```python
from build123d import *

# Parameters (mm, degrees)
SKETCH1_W            = 90
SKETCH1_H            = 120
BOSS_EXTRUDE1_DEPTH  = 15
SKETCH2_W            = 46
SKETCH2_H            = 30
CUT_EXTRUDE1_DEPTH   = 12
SKETCH3_W            = 44
SKETCH3_H            = 30
CUT_EXTRUDE2_DEPTH   = 8
SHELL1_START         = -47.6
SHELL1_OUTLINE_W     = 85.2
SHELL1_OUTLINE_H     = 13
SHELL1_DEPTH         = 45.2
SHELL1_START_2       = -117.6
SHELL1_2_OUTLINE_W   = 85.2
SHELL1_2_OUTLINE_H   = 5
SHELL1_2_DEPTH       = 35.2
SKETCH7_W            = 39
SKETCH7_H            = 34.8
CUT_EXTRUDE6_DEPTH   = 5
SKETCH11_W           = 42.056152249
SKETCH11_H           = 30
CUT_EXTRUDE9_DEPTH   = 2
CUT_EXTRUDE7_DEPTH   = 10
CUT_EXTRUDE10_DEPTH  = 3
SKETCH14_W           = 90
SKETCH14_H           = 120
SKETCH14_W_2         = 88.2
SKETCH14_H_2         = 118.2
BOSS_EXTRUDE2_DEPTH  = 1
SKETCH22_W           = 4
SKETCH22_H           = 30
BOSS_EXTRUDE6_DEPTH  = 8
SKETCH26_W           = 4
SKETCH26_H           = 12
CUT_EXTRUDE20_DEPTH  = 3.8
SKETCH27_R           = 1
CUT_EXTRUDE21_DEPTH  = 3
BOSS_EXTRUDE9_DEPTH  = 1.5
SKETCH40_R           = 3.5
CUT_EXTRUDE24_DEPTH  = 5
FILLET1_R            = 3
SKETCH44_W           = 85.2
SKETCH44_H           = 35.2
CUT_EXTRUDE25_DEPTH  = 7.8
SKETCH46_W           = 4.8
SKETCH46_H           = 15.6
BOSS_EXTRUDE15_DEPTH = 12.5
SKETCH6_R            = 0.9
CUT_EXTRUDE26_DEPTH  = 29.4
SKETCH47_W           = 33.8
SKETCH47_H           = 8
SKETCH47_W_2         = 8
BOSS_EXTRUDE16_DEPTH = 12.5
SKETCH49_W           = 41.022368698
SKETCH49_H           = 10
SKETCH49_W_2         = 8
BOSS_EXTRUDE17_DEPTH = 12.7
SKETCH50_W           = 22
SKETCH50_H           = 7
SKETCH50_W_2         = 20
SKETCH50_H_2         = 9
CUT_EXTRUDE28_DEPTH  = 12.5
FILLET3_R            = 5
FILLET4_R            = 2
SKETCH51_R           = 2.5
CUT_EXTRUDE29_DEPTH  = 6
CUT_EXTRUDE30_DEPTH  = 3
SKETCH52_R           = 1.5
CUT_EXTRUDE31_DEPTH  = 3
SKETCH54_W           = 2.470433815
SKETCH54_H           = 30
BOSS_EXTRUDE18_DEPTH = 6
SKETCH55_W           = 5
SKETCH55_H           = 2.5
CUT_EXTRUDE32_DEPTH  = 3
FILLET5_R            = 1
SKETCH56_R           = 1.25
CUT_EXTRUDE33_DEPTH  = 3
SKETCH57_W           = 2.5
SKETCH57_H           = 8
SKETCH57_W_2         = 4
BOSS_EXTRUDE19_DEPTH = 8
SKETCH58_W           = 1.5
SKETCH58_H           = 2
SKETCH58_W_2         = 2
CUT_EXTRUDE34_DEPTH  = 10
SKETCH59_W           = 9.920545957
SKETCH59_H           = 2.790153551
CUT_EXTRUDE35_DEPTH  = 10


# Read off the part's stored shape, not the designer's step: Shell1
with BuildPart() as part:
    # Sketch1 → Boss-Extrude1 (new body)
    with BuildSketch(Plane(origin=(0, 0, 0), x_dir=(1, 0, 0), z_dir=(0, 1, 0))):
        with Locations((45, 60)):
            Rectangle(SKETCH1_W, SKETCH1_H)
    extrude(amount=BOSS_EXTRUDE1_DEPTH)

    # Sketch2 → Cut-Extrude1 (cut)
    with BuildSketch(Plane(origin=(0, 15, 0), x_dir=(1, 0, 0), z_dir=(0, 1, 0))):
        with Locations((23, 65)):
            Rectangle(SKETCH2_W, SKETCH2_H)
    extrude(amount=-CUT_EXTRUDE1_DEPTH, mode=Mode.SUBTRACT)

    # Sketch3 → Cut-Extrude2 (cut)
    with BuildSketch(Plane(origin=(0, 15, 0), x_dir=(1, 0, 0), z_dir=(0, 1, 0))):
        with Locations((68, 65)):
            Rectangle(SKETCH3_W, SKETCH3_H)
    extrude(amount=-CUT_EXTRUDE2_DEPTH, mode=Mode.SUBTRACT)

    # Shell1 outline → Shell1 (cut)
    with BuildSketch(Plane.XY.offset(SHELL1_START)):
        with Locations((45, 6.5)):
            Rectangle(SHELL1_OUTLINE_W, SHELL1_OUTLINE_H)
    extrude(amount=SHELL1_DEPTH, mode=Mode.SUBTRACT)

    # Shell1 2 outline → Shell1 2 (cut)
    with BuildSketch(Plane.XY.offset(SHELL1_START_2)):
        with Locations((45, 2.5)):
            Rectangle(SHELL1_2_OUTLINE_W, SHELL1_2_OUTLINE_H)
    extrude(amount=SHELL1_2_DEPTH, mode=Mode.SUBTRACT)

    # Sketch7 → Cut-Extrude6 (cut)
    with BuildSketch(Plane.XZ):
        with Locations((68.1, -65)):
            Rectangle(SKETCH7_W, SKETCH7_H)
    extrude(amount=-CUT_EXTRUDE6_DEPTH, mode=Mode.SUBTRACT)

    # Sketch11 → Cut-Extrude9 (cut)
    with BuildSketch(Plane(origin=(0, 3, 0), x_dir=(1, 0, 0), z_dir=(0, 1, 0))):
        with Locations((24.971923875, 65)):
            Rectangle(SKETCH11_W, SKETCH11_H)
    extrude(amount=-CUT_EXTRUDE9_DEPTH, mode=Mode.SUBTRACT)

    # Sketch8 → Cut-Extrude7 (cut)
    with BuildSketch(Plane.ZY.offset(-46)):
        Polygon((-63, 1), (-63, 2.5), (-75, 2.5), (-75, 4.5), (-63, 4.5), (-63, 6), (-52, 6), (-52, 4.5), (-52, 1), align=None)
    extrude(amount=-CUT_EXTRUDE7_DEPTH, mode=Mode.SUBTRACT)

    # Sketch12 → Cut-Extrude10 (cut)
    with BuildSketch(Plane(origin=(0, 7, 0), x_dir=(1, 0, 0), z_dir=(0, 1, 0))):
        Polygon((79.361885724, 68), (79.361885724, 80), (61.361885724, 80), (61.361885724, 64.5), (77.04695331, 64.5), (77.04695331, 51), (85.714801791, 51), (85.714801791, 68), align=None)
    extrude(amount=-CUT_EXTRUDE10_DEPTH, mode=Mode.SUBTRACT)

    # Sketch14 → Boss-Extrude2 (add)
    with BuildSketch(Plane.XZ):
        with Locations((45, -60)):
            Rectangle(SKETCH14_W, SKETCH14_H)
        with Locations((45, -60)):
            Rectangle(SKETCH14_W_2, SKETCH14_H_2, mode=Mode.SUBTRACT)
    extrude(amount=BOSS_EXTRUDE2_DEPTH)

    # Sketch22 → Boss-Extrude6 (add)
    with BuildSketch(Plane(origin=(0, 7, 0), x_dir=(1, 0, 0), z_dir=(0, 1, 0))):
        with Locations((88, 65)):
            Rectangle(SKETCH22_W, SKETCH22_H)
    extrude(amount=BOSS_EXTRUDE6_DEPTH)

    # Sketch26 → Cut-Extrude20 (cut)
    with BuildSketch(Plane(origin=(0, 15, 0), x_dir=(1, 0, 0), z_dir=(0, 1, 0))):
        with Locations((88, 65)):
            Rectangle(SKETCH26_W, SKETCH26_H)
    extrude(amount=-CUT_EXTRUDE20_DEPTH, mode=Mode.SUBTRACT)

    # Sketch27 → Cut-Extrude21 (cut)
    with BuildSketch(Plane(origin=(0, 11.2, 0), x_dir=(1, 0, 0), z_dir=(0, 1, 0))):
        with Locations(Location((88, 65, 0), (0, 0, 270))):
            Circle(SKETCH27_R)
    extrude(amount=-CUT_EXTRUDE21_DEPTH, mode=Mode.SUBTRACT)

    # Sketch36 → Boss-Extrude9 (add)
    with BuildSketch(Plane.XZ.offset(-5)):
        Polygon((77.04695331, -63.5), (60.361885724, -63.5), (60.361885724, -81), (80.361885724, -81), (80.361885724, -68), (79.361885724, -68), (79.361885724, -80), (61.361885724, -80), (61.361885724, -64.5), (77.04695331, -64.5), align=None)
    extrude(amount=BOSS_EXTRUDE9_DEPTH)

    # Sketch40 → Cut-Extrude24 (cut)
    with BuildSketch(Plane.ZY):
        with Locations((-105, 7)):
            Circle(SKETCH40_R)
    extrude(amount=-CUT_EXTRUDE24_DEPTH, mode=Mode.SUBTRACT)

    # Fillet1
    fillet1_edges = [part.edges().sort_by_distance(p)[0] for p in [
        (68.1, 5, -47.6),
    ]]
    fillet(fillet1_edges, radius=FILLET1_R)

    # Sketch44 → Cut-Extrude25 (cut)
    with BuildSketch(Plane.XZ.offset(-5)):
        with Locations((45, -100)):
            Rectangle(SKETCH44_W, SKETCH44_H)
    extrude(amount=-CUT_EXTRUDE25_DEPTH, mode=Mode.SUBTRACT)

    # Sketch46 → Boss-Extrude15 (add)
    with BuildSketch(Plane.XZ.offset(-12.8)):
        with Locations((51.4, -109.8)):
            Rectangle(SKETCH46_W, SKETCH46_H)
    extrude(amount=BOSS_EXTRUDE15_DEPTH)

    # Sketch6 → Cut-Extrude26 (cut)
    with BuildSketch(Plane(origin=(0, 15, 0), x_dir=(1, 0, 0), z_dir=(0, 1, 0))):
        with Locations(Location((51.75, 108, 0), (0, 0, 270))):
            Circle(SKETCH6_R)
        with Locations(Location((51.75, 104, 0), (0, 0, 270))):
            Circle(SKETCH6_R)
    extrude(amount=-CUT_EXTRUDE26_DEPTH, mode=Mode.SUBTRACT)

    # Sketch47 → Boss-Extrude16 (add)
    with BuildSketch(Plane.XZ.offset(-12.8)):
        with Locations((70.7, -113.6)):
            Rectangle(SKETCH47_W, SKETCH47_H)
        with Locations((6.4, -113.6)):
            Rectangle(SKETCH47_W_2, SKETCH47_H)
    extrude(amount=BOSS_EXTRUDE16_DEPTH)

    # Sketch49 → Boss-Extrude17 (add)
    with BuildSketch(Plane.XZ.offset(-13)):
        with Locations((67.088815651, -7.4)):
            Rectangle(SKETCH49_W, SKETCH49_H)
        with Locations((6.4, -7.4)):
            Rectangle(SKETCH49_W_2, SKETCH49_H)
    extrude(amount=BOSS_EXTRUDE17_DEPTH)

    # Sketch50 → Cut-Extrude28 (cut)
    with BuildSketch(Plane.XZ.offset(-0.3)):
        with Locations((64.8, -113.1)):
            Rectangle(SKETCH50_W, SKETCH50_H)
        with Locations((64.939802008, -7.9)):
            Rectangle(SKETCH50_W_2, SKETCH50_H_2)
    extrude(amount=-CUT_EXTRUDE28_DEPTH, mode=Mode.SUBTRACT)

    # Fillet3
    fillet3_edges = [part.edges().sort_by_distance(p)[0] for p in [
        (10.4, 6.55, -109.6),
        (10.4, 6.65, -12.4),
        (74.939802008, 6.55, -12.4),
    ]]
    fillet(fillet3_edges, radius=FILLET3_R)

    # Fillet4
    fillet4_edges = [part.edges().sort_by_distance(p)[0] for p in [
        (0, 7, -120),
        (90, 7, -120),
        (90, 7, 0),
        (0, 7, 0),
    ]]
    fillet(fillet4_edges, radius=FILLET4_R)

    # Sketch51 → Cut-Extrude29 (cut)
    with BuildSketch(Plane.XZ.offset(-0.3)):
        with Locations(Location((84.5, -114.5, 0), (0, 0, 270))):
            Circle(SKETCH51_R)
        with Locations(Location((84.5, -5.5, 0), (0, 0, 270))):
            Circle(SKETCH51_R)
        with Locations(Location((5.5, -5.5, 0), (0, 0, 270))):
            Circle(SKETCH51_R)
        with Locations(Location((5.5, -114.5, 0), (0, 0, 270))):
            Circle(SKETCH51_R)
    extrude(amount=-CUT_EXTRUDE29_DEPTH, mode=Mode.SUBTRACT)

    # Sketch53 → Cut-Extrude30 (cut)
    with BuildSketch(Plane.XZ.offset(-0.3)):
        Polygon((53.8, -102), (49, -102), (49, -110.656453849), (53.787002796, -110.656453849), align=None)
    extrude(amount=-CUT_EXTRUDE30_DEPTH, mode=Mode.SUBTRACT)

    # Sketch52 → Cut-Extrude31 (cut)
    with BuildSketch(Plane.XZ.offset(-0.3)):
        with Locations(Location((51.19, -6.828671793, 0), (0, 0, 270))):
            Circle(SKETCH52_R)
        with Locations(Location((78.9, -112.408671793, 0), (0, 0, 270))):
            Circle(SKETCH52_R)
    extrude(amount=-CUT_EXTRUDE31_DEPTH, mode=Mode.SUBTRACT)

    # Sketch54 → Boss-Extrude18 (add)
    with BuildSketch(Plane(origin=(0, 1, 0), x_dir=(1, 0, 0), z_dir=(0, 1, 0))):
        with Locations((5.179064659, 65)):
            Rectangle(SKETCH54_W, SKETCH54_H)
    extrude(amount=BOSS_EXTRUDE18_DEPTH)

    # Sketch55 → Cut-Extrude32 (cut)
    with BuildSketch(Plane.ZY.offset(-3.943847751)):
        with Locations((-73.5, 4.75)):
            Rectangle(SKETCH55_W, SKETCH55_H)
        with Locations((-56.5, 4.75)):
            Rectangle(SKETCH55_W, SKETCH55_H)
    extrude(amount=-CUT_EXTRUDE32_DEPTH, mode=Mode.SUBTRACT)

    # Fillet5
    fillet5_edges = [part.edges().sort_by_distance(p)[0] for p in [
        (25.5, 0, -82.4),
        (25.5, 0, -47.6),
    ]]
    fillet(fillet5_edges, radius=FILLET5_R)

    # Sketch56 → Cut-Extrude33 (cut)
    with BuildSketch(Plane(origin=(0, 15, 0), x_dir=(1, 0, 0), z_dir=(0, 1, 0))):
        with Locations(Location((7, 88, 0), (0, 0, 270))):
            Circle(SKETCH56_R)
        with Locations(Location((15, 88, 0), (0, 0, 270))):
            Circle(SKETCH56_R)
        with Locations(Location((23, 88, 0), (0, 0, 270))):
            Circle(SKETCH56_R)
        with Locations(Location((31, 88, 0), (0, 0, 270))):
            Circle(SKETCH56_R)
        with Locations(Location((39, 88, 0), (0, 0, 270))):
            Circle(SKETCH56_R)
    extrude(amount=-CUT_EXTRUDE33_DEPTH, mode=Mode.SUBTRACT)

    # Sketch57 → Boss-Extrude19 (add)
    with BuildSketch(Plane.XZ.offset(-12.8)):
        with Locations((3.65, -88.4)):
            Rectangle(SKETCH57_W, SKETCH57_H)
        with Locations((45.9, -88.4)):
            Rectangle(SKETCH57_W_2, SKETCH57_H)
    extrude(amount=BOSS_EXTRUDE19_DEPTH)

    # Sketch58 → Cut-Extrude34 (cut)
    with BuildSketch(Plane(origin=(0, 0, -92.4), x_dir=(-1, 0, 0), z_dir=(0, 0, -1))):
        with Locations((-4.15, 7.3)):
            Rectangle(SKETCH58_W, SKETCH58_H)
        with Locations((-44.9, 7.3)):
            Rectangle(SKETCH58_W_2, SKETCH58_H)
    extrude(amount=-CUT_EXTRUDE34_DEPTH, mode=Mode.SUBTRACT)

    # Sketch59 → Cut-Extrude35 (cut)
    with BuildSketch(Plane(origin=(0, 15, 0), x_dir=(1, 0, 0), z_dir=(0, 1, 0))):
        with Locations((58.533039989, 112.870908725)):
            Rectangle(SKETCH59_W, SKETCH59_H)
    extrude(amount=-CUT_EXTRUDE35_DEPTH, mode=Mode.SUBTRACT)


solid = part.part
```
Design review of the part built by this model. Coordinates are the model's own, in mm. A direction names the side the tool comes from. Coordinates: 2 decimals unless noted, no trailing zeros. Loops run counter-clockwise (first coordinate to the right, second up) from the corner with the lowest first, then second, coordinate; pieces in that order, holes last. Notation, with made-up numbers: (42.25, -6) - (88.25, -6) arc R15 ccw to (88.25, 15) - close; hole circle Ø7 at (58, 38.25). An arc over 180 degrees is marked (long way). Use CSV: the item, a comma, the result in double quotes. Start each with the question number.
1) Consider section B-B on x = 23. Write out the cut boundary in (y, z), then the cut area to 3 significant figures.
2) Consider section A-A on z = -78.5. Write out the cut boundary in (x, y).
3) Consider section C-C on z = -55.5. Give the number of separate pieces and of enclosed holes in the cut face, then the cut area to 3 significant figures.
4) Wall thickness on L1, parallel to Z at x = 40, y = 8.5; L2, parallel to X at y = 1.8, z = -114.5; L3, parallel to X at y = 2.5, z = -79.5: over which ranges is each line inside the solid? List them lowest first. Write a range as from..to.
5) Tool access review of faces 1 (the flat face through (6, 6.3, -114)), 2 (the flat face through (6.414, 4, -65)), 3 (the flat face through (47, 4.5, -69)): name each direction out of +Z, -Z, +X, -X, +Y, -Y from which nothing blocks a thin tool from reaching the whole face with its end or side.
6) For pin 1 Ø2 at (x, z) = (7, -88) entering from +Y; pin 2 Ø1.2 at (x, z) = (46.5, -89) entering from -Y; pin 3 Ø5 at (x, z) = (64.5, -6.5) entering from -Y; pin 4 Ø2 at (y, z) = (6.5, -59.5) entering from -X, all flat-tipped, find the tip position at first contact; note any pin that passes through.
7) The part is to be moulded in two halves that separate along X. For faces 4 (the flat face through (53.573, 10, -113)), 5 (the flat face through (5, 5, -54)), 6 (the flat face through (90, 7, -59)), say which applies: +X half, -X half, draft (parallel to the pull), parting line (faces both ways), or undercut.
8) Consider section D-D on x = 33.5. Write out the cut boundary in (y, z).
Geometry says:
1,outline,"(-1, -120) - (15, -120) - (15, -89.25) - (12.8, -89.25) - (12.8, -117.6) - (0, -117.6) - (0, -119.1) - (-1, -119.1) - close; (-1, -0.9) - (0, -0.9) - (0, -2.4) - (13, -2.4) - (13, -47.6) - (1, -47.6) arc R1 ccw to (0, -48.6) - (0, -81.4) arc R1 ccw to (1, -82.4) - (12.8, -82.4) - (12.8, -86.75) - (15, -86.75) - (15, -80) - (1, -80) - (1, -50) - (15, -50) - (15, 0) - (-1, 0) - close"
1,area,"338 mm^2"
2,outline,"(0, -1) - (0.9, -1) - (0.9, 0) - (48.6, 0) - (48.6, 5) - (60.36, 5) - (60.36, 3.5) - (61.36, 3.5) - (61.36, 7) - (46, 7) - (46, 1) - (6.41, 1) - (6.41, 7) - (3.94, 7) - (3.94, 3) - (0, 3) - close; (79.36, 3.5) - (80.36, 3.5) - (80.36, 5) - (87.6, 5) - (87.6, 0) - (89.1, 0) - (89.1, -1) - (90, -1) - (90, 15) - (86, 15) - (86, 7) - (79.36, 7) - close"
3,separate pieces,"4"
3,enclosed holes,"0"
3,area,"172 mm^2"
4,L1,"-120..-117.6, -82.4..-80, -50..-47.6, -2.4..0"
4,L2,"0..3, 8..10.4, 49..53.8, 75.8..82, 87..90"
4,L3,"0..6.41, 46..48.6, 87.6..90"
5,face 1,"-Y"
5,face 2,"+Y"
5,face 3,"none"
6,pin 1,"through"
6,pin 2,"y = 4.8"
6,pin 3,"y = 12.8"
6,pin 4,"x = 3.94"
7,face 4,"undercut"
7,face 5,"draft"
7,face 6,"+X half"
8,outline,"(-1, -120) - (15, -120) - (15, -80) - (1, -80) - (1, -50) - (15, -50) - (15, 0) - (-1, 0) - (-1, -0.9) - (0, -0.9) - (0, -2.4) - (13, -2.4) - (13, -47.6) - (1, -47.6) arc R1 ccw to (0, -48.6) - (0, -81.4) arc R1 ccw to (1, -82.4) - (12.8, -82.4) - (12.8, -117.6) - (0, -117.6) - (0, -119.1) - (-1, -119.1) - close"
